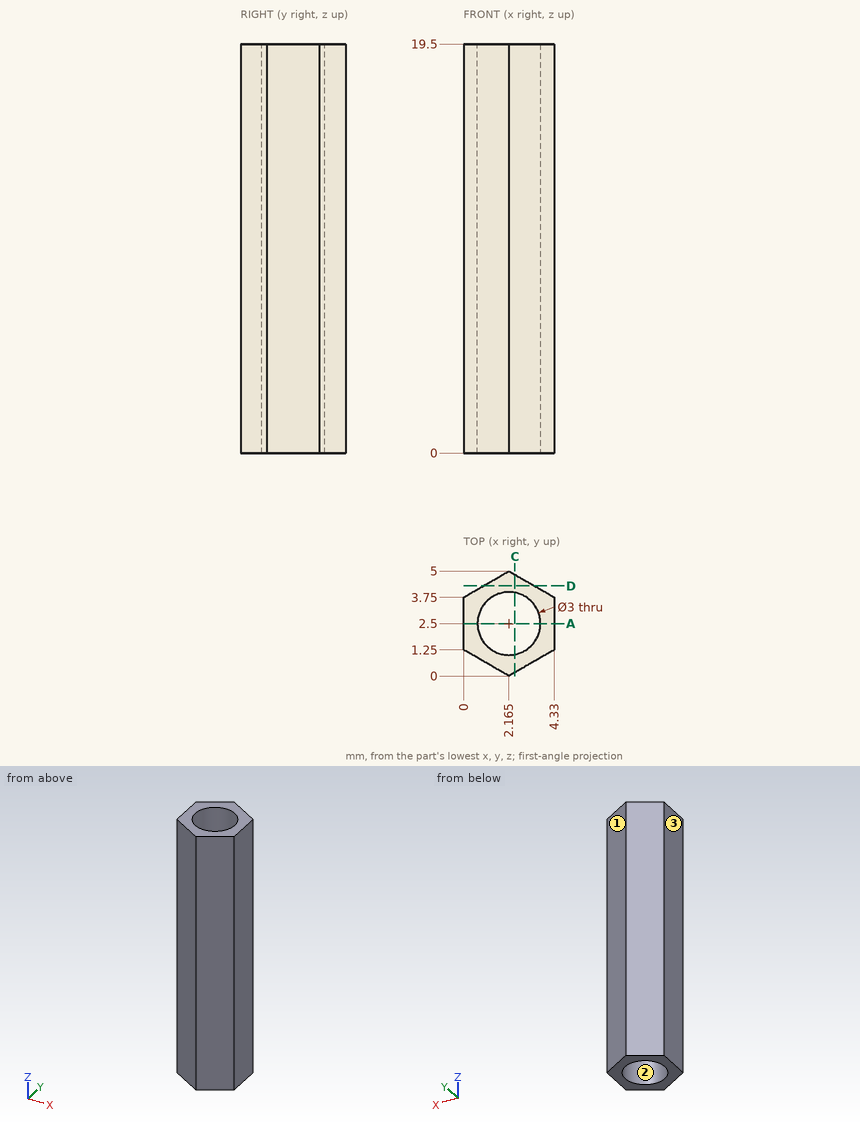
Check sheet for the drawn part. Datum: minimum x, y, z corner. Units: mm. Coordinates: 2 decimals unless noted, no trailing zeros. Loops run counter-clockwise (first coordinate to the right, second up) from the corner with the lowest first, then second, coordinate; pieces in that order, holes last. Notation, with made-up numbers: (-10.5, 83) -> (6.5, 83) arc R29 cw to (6.5, 106) -> close; hole circle Ø9 at (-32, -9.5). An arc over 180 degrees is marked (long way). Answer in a Markdown table with one row per item.
1. Sectioned sample at C-C, the plane x = 2.45. Record the boundary of the cut face in (y, z).
Check values:
| item | result |
|---|---|
| outline | (0.16, 0) -> (1.03, 0) -> (1.03, 19.5) -> (0.16, 19.5) -> close; (3.97, 0) -> (4.84, 0) -> (4.84, 19.5) -> (3.97, 19.5) -> close |
2. Sectioned sample at D-D, the plane y = 4.3. Record the boundary of the cut face in (x, z).
Check values:
| item | result |
|---|---|
| outline | (0.95, 0) -> (3.38, 0) -> (3.38, 19.5) -> (0.95, 19.5) -> close |
3. Release check for a two-part mould opening along Y. For the marked faces 1, 2 and 3 record: released by +Y, released by -Y, zero draft, split by the parting line, or undercut.
Check values:
| item | result |
|---|---|
| face 1 | released by +Y |
| face 2 | undercut |
| face 3 | zero draft |
4. Material ranges on line 1 along Y through (x, z) = (2.55, 3.25); line 2 along Y through (x, z) = (1.15, 12) (1 decimal); line 3 along X through (y, z) = (3.5, 17), recorded low to high. Write a range as [from, to].
Check values:
| item | result |
|---|---|
| line 1 | y = [0.22, 1.05], [3.95, 4.78] |
| line 2 | y = [0.6, 1.4], [3.6, 4.4] |
| line 3 | x = [0, 1.05], [3.28, 4.33] |
5. Sectioned sample at A-A, the plane y = 2.5. Record the boundary of the cut face in (x, z) (1 decimal).
Check values:
| item | result |
|---|---|
| outline | (0, 0) -> (0.7, 0) -> (0.7, 19.5) -> (0, 19.5) -> close; (3.7, 0) -> (4.3, 0) -> (4.3, 19.5) -> (3.7, 19.5) -> close |
